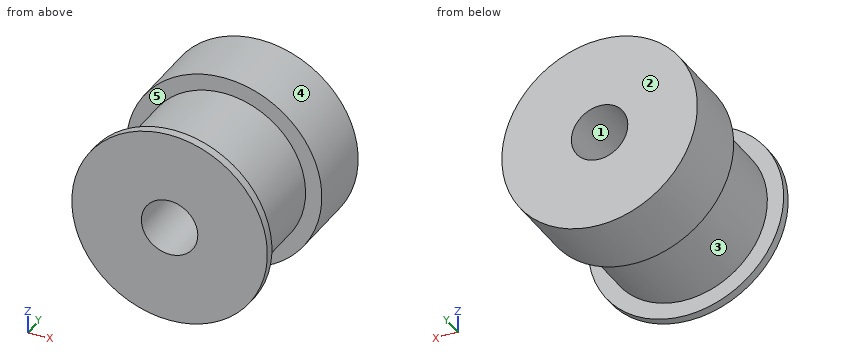
```python
from build123d import *

# Parameters (mm, degrees)
SKETCH_1_R          = 11
EXTRUDE_1_DEPTH     = 1
SKETCH_2_R          = 9.17
EXTRUDE_2_DEPTH     = 11
SKETCH_3_R          = 11
EXTRUDE_3_DEPTH     = 8
SKETCH_4_R          = 3.175
CUT_EXTRUDE_1_DEPTH = 26.337718919


with BuildPart() as part:
    # Эскиз1 → Бобышка-Вытянуть1 (new body)
    with BuildSketch(Plane(origin=(0, 0, 0), x_dir=(1, 0, 0), z_dir=(0, 1, 0))):
        with Locations(Location((0, 0, 0), (0, 0, 270))):
            Circle(SKETCH_1_R)
    extrude(amount=EXTRUDE_1_DEPTH)

    # Эскиз2 → Бобышка-Вытянуть2 (add)
    with BuildSketch(Plane(origin=(0, 1, 0), x_dir=(1, 0, 0), z_dir=(0, 1, 0))):
        with Locations(Location((0, 0, 0), (0, 0, 270))):
            Circle(SKETCH_2_R)
    extrude(amount=EXTRUDE_2_DEPTH)

    # Эскиз3 → Бобышка-Вытянуть3 (add)
    with BuildSketch(Plane(origin=(0, 12, 0), x_dir=(1, 0, 0), z_dir=(0, 1, 0))):
        with Locations(Location((0, 0, 0), (0, 0, 270))):
            Circle(SKETCH_3_R)
    extrude(amount=EXTRUDE_3_DEPTH)

    # Эскиз4 → Вырез-Вытянуть1 (cut, through all)
    with BuildSketch(Plane(origin=(0, 20, 0), x_dir=(1, 0, 0), z_dir=(0, 1, 0))):
        with Locations(Location((0, 0, 0), (0, 0, 270))):
            Circle(SKETCH_4_R)
    extrude(amount=-CUT_EXTRUDE_1_DEPTH, mode=Mode.SUBTRACT)


solid = part.part
```
Read the model definition and answer for the solid it produces. Units are mm, in the model's axes. Face numbers are marked on the shaded views. A direction names the side the tool comes from. Coordinates: 2 decimals unless noted, no trailing zeros. Write each loop counter-clockwise with the first axis right and the second up, starting at its lowest first coordinate (ties: lowest second). Pieces come first, ordered by that corner, then holes. Notation, with made-up numbers: (12, -37) -> (55, -37) arc R24 cw to (55, -9) -> close; hole circle Ø3 at (78.5, 32.5). An arc over 180 degrees is marked (long way). Answer as a JSON object with one key per item and string values.
Q1. The part is cut by section B-B on x = 0. Give the vertices of the cut face in (y, z) (3 decimals), then the cut area to 3 significant figures.
The answers:
{"outline": "(0, -11) -> (1, -11) -> (1, -9.17) -> (12, -9.17) -> (12, -11) -> (20, -11) -> (20, -3.175) -> (0, -3.175) -> close; (0, 3.175) -> (20, 3.175) -> (20, 11) -> (12, 11) -> (12, 9.17) -> (1, 9.17) -> (1, 11) -> (0, 11) -> close", "area": "273 mm2"}
Q2. Flat-ended cylindrical pins translate along their axes: pin 1 Ø4 at (x, y) = (7, 9) entering from -Z; pin 2 Ø3 at (x, y) = (-2, 10) entering from -Z; pin 3 Ø5 at (x, y) = (-6, 16.5) entering from +Z. Find the tip coordinate at first contact, or state that the pin passes through.
The answers:
{"pin 1": "stops at z = -7.69", "pin 2": "stops at z = -9.16", "pin 3": "stops at z = 10.43"}
Q3. The part is cut by section A-A on z = 0. Give the vertices of the cut face in (x, y) (3 decimals).
The answers:
{"outline": "(-11, 0) -> (-3.175, 0) -> (-3.175, 20) -> (-11, 20) -> (-11, 12) -> (-9.17, 12) -> (-9.17, 1) -> (-11, 1) -> close; (3.175, 0) -> (11, 0) -> (11, 1) -> (9.17, 1) -> (9.17, 12) -> (11, 12) -> (11, 20) -> (3.175, 20) -> close"}
Q4. A tool of negligible diameter and unlimited length cuts with its end or side. For the marked faces 4 and 5, from which of +Z, -Z, +X, -X, +Y, -Y can it reach the whole face along a straight path? Write none if from no direction.
The answers:
{"face 4": "+Y, -Y", "face 5": "none"}
Q5. The part is cut by section D-D on z = -7.5. Give the vertices of the cut face in (x, y), then the cut area to 3 significant figures.
The answers:
{"outline": "(-8.05, 0) -> (8.05, 0) -> (8.05, 1) -> (5.28, 1) -> (5.28, 12) -> (8.05, 12) -> (8.05, 20) -> (-8.05, 20) -> (-8.05, 12) -> (-5.28, 12) -> (-5.28, 1) -> (-8.05, 1) -> close", "area": "261 mm2"}
Q6. Determine the mould class of the marked faces 1, 2 and 3 for opening direction Z: pulls with the +Z half, pulls with the -Z half, needs draft (parallel to the pull), parting line crosses it, or undercut.
The answers:
{"face 1": "undercut", "face 2": "needs draft", "face 3": "parting line crosses it"}
Q7. The part is cut by section C-C on y = 16. Give the vertices of the cut face in (x, z) (3 decimals).
The answers:
{"outline": "circle Ø22 at (0, 0); hole circle Ø6.35 at (0, 0)"}
Q8. Consider line 1 (X direction, y = 5, z = 0) (3 decimals); line 2 (Y direction, x = -8.25, z = -6); line 3 (X direction, y = 13.25, z = 0) (3 decimals). Determine where each line is inside the solid, lowest interval first. Write a range as [from, to].
The answers:
{"line 1": "x = [-9.17, -3.175], [3.175, 9.17]", "line 2": "y = [0, 1], [12, 20]", "line 3": "x = [-11, -3.175], [3.175, 11]"}
